Geometry check sheet. Reference: the model listing, model coordinates, mm. Face numbers are marked on the shaded views. A direction names the side the tool comes from. Coordinates: 2 decimals unless noted, no trailing zeros. Loops run counter-clockwise (first coordinate to the right, second up) from the corner with the lowest first, then second, coordinate; pieces in that order, holes last.
from build123d import *

# Parameters (mm, degrees)
SKETCH1_R           = 10
BOSS_EXTRUDE1_DEPTH = 100
SKETCH2_R           = 12.5
BOSS_EXTRUDE2_DEPTH = 10
SKETCH3_R           = 9.5
BOSS_EXTRUDE3_DEPTH = 7
SKETCH4_R           = 6
BOSS_EXTRUDE4_DEPTH = 6
SKETCH5_R           = 9.5
BOSS_EXTRUDE5_DEPTH = 7
SKETCH6_W           = 5
SKETCH6_H           = 6
CUT_EXTRUDE1_DEPTH  = 20


with BuildPart() as part:
    # Sketch1 → Boss-Extrude1 (new body)
    with BuildSketch(Plane.XY):
        Circle(SKETCH1_R)
    extrude(amount=BOSS_EXTRUDE1_DEPTH)

    # Sketch2 → Boss-Extrude2 (add)
    with BuildSketch(Plane.XY.offset(100)):
        Circle(SKETCH2_R)
    extrude(amount=BOSS_EXTRUDE2_DEPTH)

    # Sketch3 → Boss-Extrude3 (add)
    with BuildSketch(Plane.XY.offset(110)):
        Circle(SKETCH3_R)
    extrude(amount=BOSS_EXTRUDE3_DEPTH)

    # Sketch4 → Boss-Extrude4 (add)
    with BuildSketch(Plane.XY.offset(117)):
        Circle(SKETCH4_R)
    extrude(amount=BOSS_EXTRUDE4_DEPTH)

    # Sketch5 → Boss-Extrude5 (add)
    with BuildSketch(Plane.XY.offset(123)):
        Circle(SKETCH5_R)
    extrude(amount=BOSS_EXTRUDE5_DEPTH)

    # Sketch6 → Cut-Extrude1 (cut)
    with BuildSketch(Plane(origin=(0, 0, 0), x_dir=(-1, 0, 0), z_dir=(0, 0, -1))):
        with Locations((-9.5, 0)):
            Rectangle(SKETCH6_W, SKETCH6_H)
    extrude(amount=-CUT_EXTRUDE1_DEPTH, mode=Mode.SUBTRACT)


solid = part.part
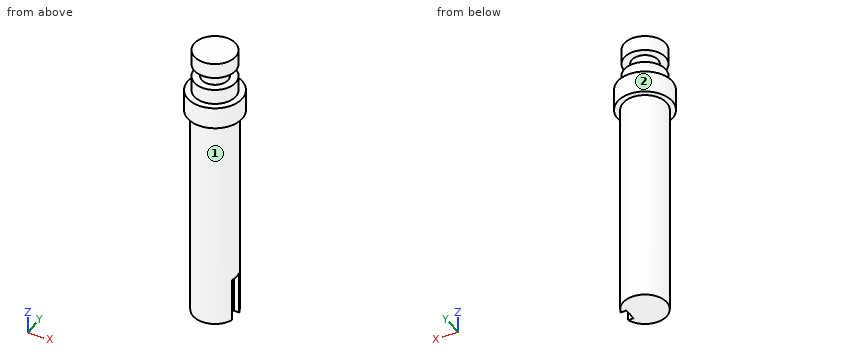
(1) Access from +Z, -Z, +X, -X, +Y, -Y to the whole of each face (thin tool, end or side, straight path). Record for the marked faces 1 and 2.
Findings:
face 1: -Z
face 2: +Z, -Z
(2) Sectioned sample at B-B on y = 0. Record the cut outline in (x, z).
Findings:
outline: (-12.5, 100) - (-10, 100) - (-10, 0) - (7, 0) - (7, 20) - (10, 20) - (10, 100) - (12.5, 100) - (12.5, 110) - (9.5, 110) - (9.5, 117) - (6, 117) - (6, 123) - (9.5, 123) - (9.5, 130) - (-9.5, 130) - (-9.5, 123) - (-6, 123) - (-6, 117) - (-9.5, 117) - (-9.5, 110) - (-12.5, 110) - close
(3) Sectioned sample at D-D on z = 120. Record the cut outline in (x, y), and give its area (3 significant figures).
Findings:
outline: circle Ø12 at (0, 0)
area: 113 mm2
(4) Scan lines: L1, parallel to Z at x = 0.25, y = -7.25; L2, parallel to X at y = -0.5, z = 34; L3, parallel to Z at x = 3, y = 11. Record each from-to range of solid material in increasing order.
Findings:
L1: z = 0 to 117, 123 to 130
L2: x = -9.99 to 9.99
L3: z = 100 to 110
(5) Sectioned sample at A-A on x = 0. Record the cut outline in (y, z).
Findings:
outline: (-12.5, 100) - (-10, 100) - (-10, 0) - (10, 0) - (10, 100) - (12.5, 100) - (12.5, 110) - (9.5, 110) - (9.5, 117) - (6, 117) - (6, 123) - (9.5, 123) - (9.5, 130) - (-9.5, 130) - (-9.5, 123) - (-6, 123) - (-6, 117) - (-9.5, 117) - (-9.5, 110) - (-12.5, 110) - close
(6) Sectioned sample at C-C on z = 93.5. Record the cut outline in (x, y).
Findings:
outline: circle Ø20 at (0, 0)
(7) Gauge pin test, flat ends, axial feed: pin 1 Ø1 at (x, z) = (9, 57.5) entering from -Y; pin 2 Ø5 at (x, z) = (-6.5, 52) entering from -Y; pin 3 Ø1.3 at (x, z) = (8.5, 8.5) entering from +Y. Record the tip position at first contact, or that the pin passes through.
Findings:
pin 1: stops at y = -5.27
pin 2: stops at y = -9.17
pin 3: stops at y = 6.19
